Could you check a few things on this model? Use its own coordinates, in mm. Face numbers are marked on the shaded views. A direction names the side the tool comes from. Coordinates: 2 decimals unless noted, no trailing zeros. Loops run counter-clockwise (first coordinate to the right, second up) from the corner with the lowest first, then second, coordinate; pieces in that order, holes last. Notation, with made-up numbers: M 86,-31.75 L 141,-31.75 A21 cw 141,-7.75 Z; hole C 70.25,13.5 d7. An arc over 180 degrees is marked long. Write each question's results on one line, items separated by ' | '.
Solid Edge part; units mm, degrees
sketch "Sketch1" plane through (0, 0, 0) normal (0, 0, 1) x (1, 0, 0)
  line L0 (15, -6.5) -> (-15, -6.5)
  line L1 (-15, -6.5) -> (-15, 6.5)
  line L2 (-15, 6.5) -> (15, 6.5)
  line L3 (15, 6.5) -> (15, -6.5)
  dimension "D1" = 15
  dimension "D2" = 15
extrude "Protrusion1" add sketch "Sketch1" along normal blind 8
hole "Hole_1" at (0, 0, 8) direction (0, 0, -1) diameter 6 end through all
hole "Hole_2" at (0, -6.5, 4) direction (0, 1, 0) diameter 4 end up to next
hole "Hole_3" at (-10, 0, 8) direction (0, 0, -1) diameter 3.2 depth 140
hole "Hole1" at (10, 0, 8) direction (0, 0, -1) diameter 3.2 depth 140
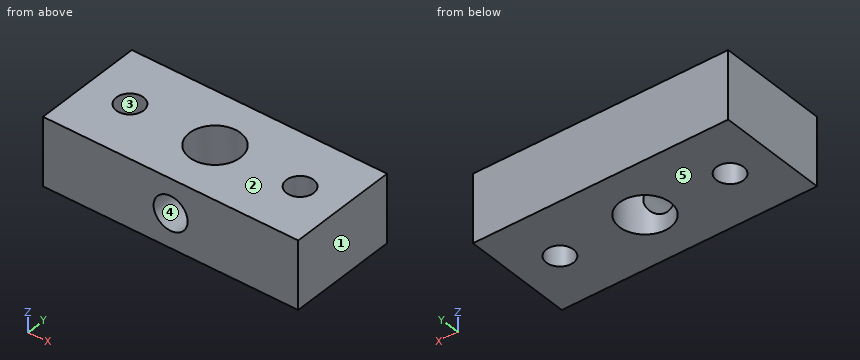
(1) Imagine slicing it at D-D, the plane z = 4. List the corners of the cut face in (x, y) for me.
Reported:
outline: M -15,-6.5 L -2,-6.5 L -2,-2.24 A3 cw long 2,-2.24 L 2,-6.5 L 15,-6.5 L 15,6.5 L -15,6.5 Z; hole C -10,0 d3.2; hole C 10,0 d3.2
(2) Which directions (+Z, -Z, +X, -X, +Y, -Y) give clear straight access to the entire face, cutting with the end or side of a thin tool? Please do the marked faces 4 and 5.
Reported:
face 4: -Y | face 5: -Z, +X, -X, +Y, -Y
(3) Imagine slicing it at A-A, the plane x = 0. List the corners of the cut face in (y, z) for me, and give its area (3 significant figures).
Reported:
outline: M -6.5,0 L -3,0 L -3,2 L -6.5,2 Z; M -6.5,6 L -3,6 L -3,8 L -6.5,8 Z; M 3,0 L 6.5,0 L 6.5,8 L 3,8 Z | area: 42.0 mm2
(4) Imagine slicing it at B-B, the plane y = 0. List the corners of the cut face in (x, z) for me, and give its area (3 significant figures).
Reported:
outline: M -15,0 L -11.6,0 L -11.6,8 L -15,8 Z; M -8.4,0 L -3,0 L -3,8 L -8.4,8 Z; M 3,0 L 8.4,0 L 8.4,8 L 3,8 Z; M 11.6,0 L 15,0 L 15,8 L 11.6,8 Z | area: 141 mm2
(5) Please list where these lines run through material, in increasing order: probe 1 along X at (y, z) = (0, 3); probe 2 along Y at (x, z) = (10, 5.25); probe 3 along X at (y, z) = (1, 7). Write a range as from..to.
Reported:
probe 1: x = -15..-11.6, -8.4..-3, 3..8.4, 11.6..15 | probe 2: y = -6.5..-1.6, 1.6..6.5 | probe 3: x = -15..-11.25, -8.75..-2.83, 2.83..8.75, 11.25..15
(6) Will this pin go through, and if not, where does the flat tip stop? P1, Ø3, axis at x = 11.5, y = -1.5, coming from the -Z side.
Reported:
P1: stops at z = 0
(7) If we mould it in two halves opening along X, with no side actions, what happens to the marked faces 1, 2 and 3? For each: released by +X, released by -X, zero draft, split by the parting line, or undercut.
Reported:
face 1: released by +X | face 2: zero draft | face 3: undercut
(8) Imagine slicing it at C-C, the plane x = 10. List the corners of the cut face in (y, z) for me, and give its area (3 significant figures).
Reported:
outline: M -6.5,0 L -1.6,0 L -1.6,8 L -6.5,8 Z; M 1.6,0 L 6.5,0 L 6.5,8 L 1.6,8 Z | area: 78.4 mm2
